```python
from build123d import *

# Parameters (mm, degrees)
BOSS_EXTRUDE1_DEPTH = 120
END_SIZE            = 1


with BuildPart() as part:
    # Sketch1 → Boss-Extrude1 (new body)
    with BuildSketch(Plane.XY):
        with BuildLine():
            Line((-16.18058706286363, 3.583270500183823), (-20.41674499500726, 6.773876394671033))
            ThreePointArc((-20.41674499500726, 6.773876394671035), (-22.889384976175005, 5.316593545441291), (-23.607350889494484, 2.5377184625273967))
            Line((-23.607350889494484, 2.5377184625273967), (-19.371192957350857, -0.6528874319598208))
            ThreePointArc((-19.371192957350857, -0.6528874319598175), (-17.06351759251198, 0.6006072959958577), (-16.14396897617906, 3.0604944813556076))
            ThreePointArc((-16.14396897617906, 3.0604944813556085), (-16.153134699247452, 3.3225229388436817), (-16.180587062863637, 3.583270500183822))
        make_face()
    extrude(amount=BOSS_EXTRUDE1_DEPTH)

    # End
    end_edges = [part.edges().sort_by_distance(p)[0] for p in [
        (-22.889384976175005, 5.316593545441292, 120),
        (-21.48927192342267, 0.9424155152837879, 120),
        (-16.89855297618315, 0.8043954172700718, 120),
        (-16.898552976183115, 0.8043954172699284, 0),
        (-18.298666028935443, 5.1785734474274285, 120),
        (-21.48927192342267, 0.9424155152837879, 0),
        (-22.889384976175005, 5.316593545441292, 0),
        (-18.298666028935443, 5.1785734474274285, 0),
    ]]
    chamfer(end_edges, length=END_SIZE)


solid = part.part
```
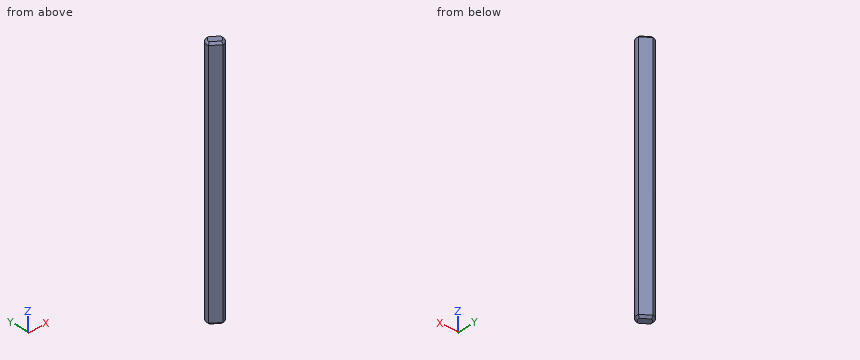
Geometry: final body of the model. Coordinates: model frame, mm. Coordinates: 2 decimals unless noted, no trailing zeros. Write each loop counter-clockwise with the first axis right and the second up, starting at its lowest first coordinate (ties: lowest second). Pieces come first, ordered by that corner, then holes. Notation, with made-up numbers: M 86.25,-32.75 L 119.25,-32.75 A24 cw 119.25,-3.75 Z; hole C 43,45.5 d2. An arc over 180 degrees is marked long. Answer as CSV lines item,"result". Start each with the question number.
Q1. Pin query (flat end, axial travel): P1, Ø2, axis at y = 1.5, z = 99, coming from the +X side; P2, Ø1, axis at x = -18, y = 5, coming from the -Z side. Return the tip coordinate at first contact, or that it passes through.
Q2. Line query: line 1 (X direction, y = 2.75, z = 74); line 2 (Y direction, x = -19, z = 33.5); line 3 (X direction, y = 2.25, z = 92). Output: solid intervals per line, ascending. Write a range as from..to.
Q3. Cut plane A-A on z = 37.5. Return the cut outline in (x, y), then the cut area to 3 significant figures.
Findings below:
1,P1,"stops at x = -16.19"
1,P2,"stops at z = 0.54"
2,line 1,"x = -23.63..-16.16"
2,line 2,"y = -0.58..5.71"
2,line 3,"x = -23.23..-16.23"
3,outline,"M -23.61,2.54 L -19.37,-0.65 A3.75 ccw -16.18,3.58 L -20.42,6.77 A3.75 ccw Z"
3,area,"36.2 mm2"
